Check sheet for the drawn part. Datum: minimum x, y, z corner. Units: mm. Round coordinates to 2 decimals unless told otherwise and drop trailing zeros. Order: outer loops, then holes, each group sorted by start corner. A loop starts at its lowest first (then second) coordinate and runs counter-clockwise, first axis right, second up. Notation, with made-up numbers: (-8.75, -26) -> (0.25, -26) arc R12 cw to (0.25, -21) -> close; hole circle Ø10 at (0, 12). An arc over 180 degrees is marked (long way). Answer in a Markdown table with one row per item.
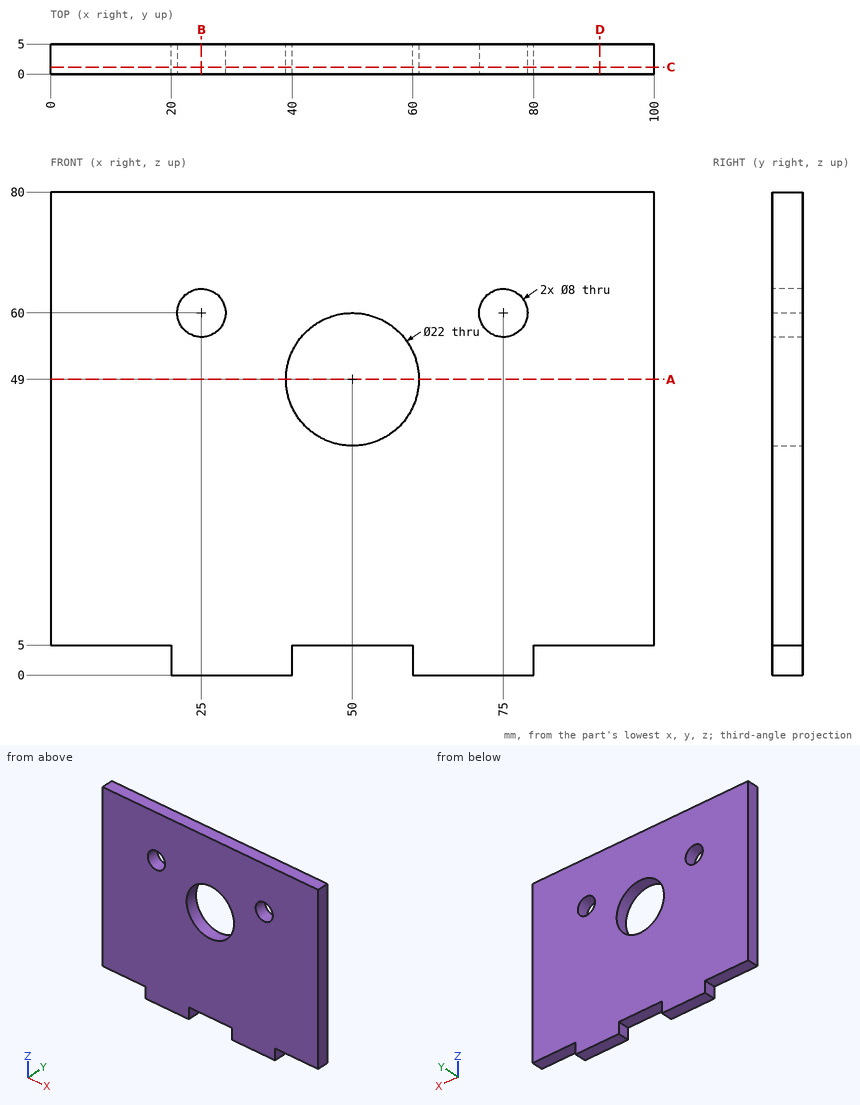
(1) Scan lines: probe 1 along Z at (x, y) = (25, 2.2); probe 2 along X at (y, z) = (3.55, 61); probe 3 along Z at (x, y) = (50, 2.7). Record each from-to range of solid material in increasing order. Write a range as from..to.
Solutions:
| item | result |
|---|---|
| probe 1 | 0..56, 64..80 |
| probe 2 | 0..21.13, 28.87..71.13, 78.87..100 |
| probe 3 | 5..38, 60..80 |
(2) Section check B-B on x = 25. Record the boundary of the cut face in (y, z), plus the area to 3 significant figures.
Solutions:
| item | result |
|---|---|
| outline | (0, 0) -> (5, 0) -> (5, 56) -> (0, 56) -> close; (0, 64) -> (5, 64) -> (5, 80) -> (0, 80) -> close |
| area | 360 mm^2 |
(3) Section check C-C on y = 1.15. Record the boundary of the cut face in (x, z), plus the area to 3 significant figures.
Solutions:
| item | result |
|---|---|
| outline | (0, 5) -> (20, 5) -> (20, 0) -> (40, 0) -> (40, 5) -> (60, 5) -> (60, 0) -> (80, 0) -> (80, 5) -> (100, 5) -> (100, 80) -> (0, 80) -> close; hole circle Ø8 at (25, 60); hole circle Ø22 at (50, 49); hole circle Ø8 at (75, 60) |
| area | 7,220 mm^2 |
(4) Section check D-D on x = 91. Record the boundary of the cut face in (y, z).
Solutions:
| item | result |
|---|---|
| outline | (0, 5) -> (5, 5) -> (5, 80) -> (0, 80) -> close |
(5) Depth check by flat-ended pin: pin 1 Ø2.5 at (y, z) = (1.5, 2.5) entering from +X; pin 2 Ø2.5 at (y, z) = (3.5, 1.5) entering from -X; pin 3 Ø1.5 at (x, y) = (12, 1.5) entering from -Z; pin 4 Ø17.5 at (x, z) = (50, 49) entering from -Y. Enter the tip coordinate at first touch or a pass-through.
Solutions:
| item | result |
|---|---|
| pin 1 | x = 80 |
| pin 2 | x = 20 |
| pin 3 | z = 5 |
| pin 4 | through |
(6) Section check A-A on z = 49. Record the boundary of the cut face in (x, y), plus the area to 3 significant figures.
Solutions:
| item | result |
|---|---|
| outline | (0, 0) -> (39, 0) -> (39, 5) -> (0, 5) -> close; (61, 0) -> (100, 0) -> (100, 5) -> (61, 5) -> close |
| area | 390 mm^2 |
